from build123d import *

# Parameters (mm, degrees)
SKETCH1_R           = 1.27
BOSS_EXTRUDE1_DEPTH = 3.81
FILLET1_R           = 8.128
FILLET2_R           = 5.588
FILLET3_R           = 2.54
FILLET4_R           = 2.54


with BuildPart() as part:
    # Sketch1 → Boss-Extrude1 (new body)
    with BuildSketch(Plane(origin=(0, 0, 0), x_dir=(1, 0, 0), z_dir=(0, 1, 0))):
        Polygon((26.917778839, 57.028322157), (18.764761653, 58.551267753), (19.231154767, 61.048081215), (-4.411826254, 65.464479834), (-4.878219367, 62.967666372), (-13.031236553, 64.490611968), (-22.811913306, 61.740346117), (-23.499479769, 64.185515305), (-43.060833275, 58.684983602), (-42.373266812, 56.239814414), (-52.153943565, 53.489548563), (-56.864625449, 44.487600096), (-59.115112565, 45.665270567), (-68.536476333, 27.661373635), (-66.285989216, 26.483703164), (-70.9966711, 17.481754697), (-45.779512683, -24.409388032), (29.596058622, -24.409388032), (29.864982666, -14.252947718), (32.404982666, -14.320202292), (32.942830753, 5.992678337), (30.402830753, 6.059932911), (30.671754796, 16.216373225), (48.398722953, 22.529356376), (43.028486925, 31.154097821), (45.184672286, 32.496656828), (34.444200229, 49.746139719), (32.288014868, 48.403580712), align=None)
        with Locations(Location((28.652499761, -12.063891898, 0), (0, 0, 90))):
            Circle(SKETCH1_R, mode=Mode.SUBTRACT)
        with Locations(Location((29.076203579, 3.938108102, 0), (0, 0, 90))):
            Circle(SKETCH1_R, mode=Mode.SUBTRACT)
        with Locations(Location((-64.159725757, 27.807781977, 0), (0, 0, 90))):
            Circle(SKETCH1_R, mode=Mode.SUBTRACT)
        with Locations(Location((-56.740401791, 41.985850812, 0), (0, 0, 90))):
            Circle(SKETCH1_R, mode=Mode.SUBTRACT)
        with Locations(Location((-39.951089771, 55.601661313, 0), (0, 0, 90))):
            Circle(SKETCH1_R, mode=Mode.SUBTRACT)
        with Locations(Location((-24.546523885, 59.933330029, 0), (0, 0, 90))):
            Circle(SKETCH1_R, mode=Mode.SUBTRACT)
        with Locations(Location((40.809219088, 32.315575875, 0), (0, 0, 90))):
            Circle(SKETCH1_R, mode=Mode.SUBTRACT)
        with Locations(Location((-1.154887819, 60.980198638, 0), (0, 0, 90))):
            Circle(SKETCH1_R, mode=Mode.SUBTRACT)
        with Locations(Location((14.575036992, 58.041922025, 0), (0, 0, 90))):
            Circle(SKETCH1_R, mode=Mode.SUBTRACT)
        with Locations(Location((32.351097343, 45.899543651, 0), (0, 0, 90))):
            Circle(SKETCH1_R, mode=Mode.SUBTRACT)
    extrude(amount=BOSS_EXTRUDE1_DEPTH)

    # Fillet1
    fillet1_edges = [part.edges().sort_by_distance(p)[0] for p in [
        (29.596058622, 1.905, 24.409388032),
        (-45.779512683, 1.905, 24.409388032),
        (-70.9966711, 1.905, -17.481754697),
        (-52.153943565, 1.905, -53.489548563),
        (-13.031236553, 1.905, -64.490611968),
        (26.917778839, 1.905, -57.028322157),
        (48.398722953, 1.905, -22.529356376),
    ]]
    fillet(fillet1_edges, radius=FILLET1_R)

    # Fillet2
    fillet2_edges = [part.edges().sort_by_distance(p)[0] for p in [
        (30.671754796, 1.905, -16.216373225),
    ]]
    fillet(fillet2_edges, radius=FILLET2_R)

    # Fillet3
    # the kernel refuses this fillet: 2.54 mm, written as the material it adds along each edge
    with BuildSketch(Plane(origin=(43.028486925, 0, -31.154097821), x_dir=(0.42954622715766955, 0, 0.9030448708312405), z_dir=(0, 1, 0))) as fillet3_piece_1:
        with BuildLine():
            CenterArc((2.27034081, 2.521441091), FILLET3_R, 186.469886636, 76.599657859)
            Line((-0.253482478, 2.235231353), (-0.505864807, 2.206610379))
            Line((-0.505864807, 2.206610379), (-0.252382329, -0.028620974))
            Line((-0.252382329, -0.028620974), (0.028620974, -0.252382329))
            ThreePointArc((0.028620974, -0.252382329), (0.095841513, -0.244759302), (1.933204138, -0.252144109))
            Line((1.933204138, -0.252144109), (1.963852927, 0))
        make_face()
    extrude(amount=3.81)
    with BuildSketch(Plane(origin=(29.864982666, 0, 14.252947718), x_dir=(0.9996496372388306, 0, 0.02646890190911047), z_dir=(0, 1, 0))) as fillet3_piece_2:
        with BuildLine():
            CenterArc((2.535902872, -2.54), FILLET3_R, 90, 88.412002671)
            Line((-0.003121621, -2.469610926), (-0.25702407, -2.462572019))
            ThreePointArc((-0.25702407, -2.462572019), (-0.254, -2.244365891), (-0.254, 0))
            Line((-0.254, 0), (0, 0.254))
            Line((0, 0.254), (2.535902872, 0.254))
            Line((2.535902872, 0.254), (2.535902872, 0))
        make_face()
    extrude(amount=3.81)
    with BuildSketch(Plane(origin=(30.402830753, 0, -6.059932911), x_dir=(0.026468901909109464, 0, -0.9996496372388307), z_dir=(0, 1, 0)), Plane(origin=(-66.285989216, 0, -26.483703164), x_dir=(-0.4636497916963805, 0, 0.8860185498396199), z_dir=(0, 1, 0)), Plane(origin=(-56.864625449, 0, -44.487600096), x_dir=(-0.8860185498396245, 0, -0.46364979169637166), z_dir=(0, 1, 0))) as fillet3_piece_3:
        with BuildLine():
            CenterArc((FILLET3_R, -FILLET3_R), FILLET3_R, 90, 90)
            Line((0, -FILLET3_R), (0, 0))
            Line((0, 0), (FILLET3_R, 0))
        make_face()
    extrude(amount=3.81)
    with BuildSketch(Plane(origin=(-42.373266812, 0, -56.239814414), x_dir=(-0.27069545780340803, 0, -0.9626650347470834), z_dir=(0, 1, 0)), Plane(origin=(-22.811913306, 0, -61.740346117), x_dir=(0.9626650347470831, 0, -0.27069545780340953), z_dir=(0, 1, 0)), Plane(origin=(-4.878219367, 0, -62.967666372), x_dir=(0.18361933590472898, 0, -0.9829974259792882), z_dir=(0, 1, 0)), Plane(origin=(18.764761653, 0, -58.551267753), x_dir=(0.9829974259792874, 0, 0.18361933590473364), z_dir=(0, 1, 0)), Plane(origin=(32.288014868, 0, -48.403580712), x_dir=(0.848891874527916, 0, -0.5285665382527359), z_dir=(0, 1, 0))) as fillet3_piece_4:
        with BuildLine():
            CenterArc((FILLET3_R, FILLET3_R), FILLET3_R, 180, 90)
            Line((0, FILLET3_R), (0, 0))
            Line((0, 0), (FILLET3_R, 0))
        make_face()
    extrude(amount=3.81)

    # Fillet4
    fillet4_edges = [part.edges().sort_by_distance(p)[0] for p in [
        (32.404982666, 1.905, 14.320202292),
        (32.942830753, 1.905, -5.992678337),
        (45.184672286, 1.905, -32.496656828),
        (34.444200229, 1.905, -49.746139719),
        (19.231154767, 1.905, -61.048081215),
        (-4.411826254, 1.905, -65.464479834),
        (-23.499479769, 1.905, -64.185515305),
        (-43.060833275, 1.905, -58.684983602),
        (-59.115112565, 1.905, -45.665270567),
        (-68.536476333, 1.905, -27.661373635),
    ]]
    fillet(fillet4_edges, radius=FILLET4_R)


solid = part.part
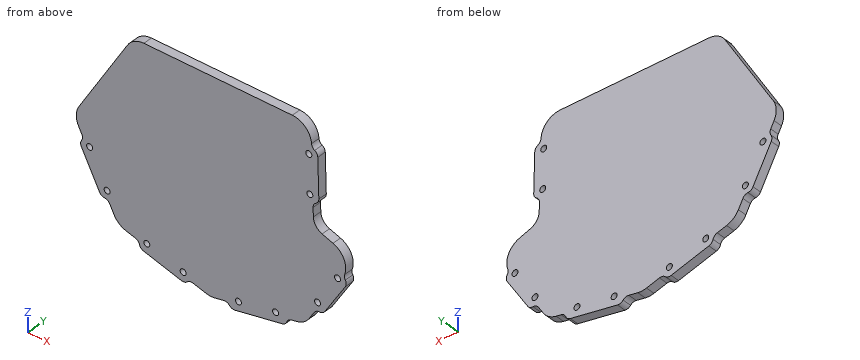
Geometry check sheet. Reference: the model listing, model coordinates, mm. Give positions to 0.01 mm unless a question says otherwise; leave off trailing zeros. Order: outer loops, then holes, each group sorted by start corner. A loop starts at its lowest first (then second) coordinate and runs counter-clockwise, first axis right, second up.
1) Material ranges on probe 1 along X at (y, z) = (1.2, -59); probe 2 along X at (y, z) = (1.3, 12.5); probe 3 along Z at (x, y) = (-40.5, 0.55), recorded low to high.
Results are:
probe 1: x = -41.75 to -25.41, -23.69 to 13.74, 15.41 to 19.74
probe 2: x = -52.95 to 27.46, 29.85 to 32.45
probe 3: z = -59.41 to -56.75, -54.46 to 24.41
2) Cross-section at B-B (z = -52). Record the boundary of the cut face in (x, y), then the cut area to 3 significant figures.
Results are:
outline: (-52.67, 0) - (30.05, 0) - (30.05, 3.81) - (-52.67, 3.81) - close
area: 315 mm2
3) Gauge pin test, flat ends, axial feed: pin 1 (2 mm diameter, centred on y = 3, z = -21, fed in from +X); pin 2 (1.5 mm diameter, centred on x = -51, y = 1.5, fed in from +Z). Record the tip position at first contact, or that the pin passes through.
Results are:
pin 1: stops at x = 42.72
pin 2: stops at z = 16.98
4) Cross-section at A-A (y = 2.8). Give the number of separate pieces and of enclosed holes in the cut face, then the cut area to 3 significant figures.
Results are:
separate pieces: 1
enclosed holes: 10
area: 8,030 mm2
5) Cross-section at C-C (z = 18). Record the boundary of the cut face in (x, y).
Results are:
outline: (-49.64, 0) - (29.62, 0) - (29.62, 3.81) - (-49.64, 3.81) - close
